Design review of the part built by this model. Coordinates are the model's own, in mm. A direction names the side the tool comes from. Coordinates: 2 decimals unless noted, no trailing zeros. Write each loop counter-clockwise with the first axis right and the second up, starting at its lowest first coordinate (ties: lowest second). Pieces come first, ordered by that corner, then holes.
Q1. Take a section at C-C (x = 5). Give the boundary of the cut face in (y, z).
Q2. Mouldability with a two-part tool opening along X and no side actions: class faces 6 (the flat face through (6.25, 0, 45)), 7 (the flat face through (10, 7, 13)), 8 (the flat face through (-19, 0, 30)), 9 (the flat face through (-7, 0, 12)) as pulls with the +X half, pulls with the -X half, needs draft (parallel to the pull), parting line crosses it, or undercut.
Q3. For probe 1 along X at (y, z) = (0, 24); probe 2 along Z at (x, y) = (4, 6); probe 3 along Y at (x, z) = (-3, 45), list the stretches that pass through material, from the lowest coordinate up.
Q4. Machinability: for faces 1 (the flat face through (19, 0, 30)), 2 (the flat face through (-25, 0, 35)), 3 (the flat face through (-6.25, 0, 45)), 4 (the flat face through (-11, 7, 12)), 5 (the flat face through (0, 3.5, 45)), which of the approach directions +Z, -Z, +X, -X, +Y, -Y give a long, thin tool a straight path to every point of the face, cutting with its end or side? Answer none if there is none.
Q5. Insertion check: pin 1 (6 mm diameter, centred on y = 1.5, z = 24.5, fed in from -X); pin 2 (7 mm diameter, centred on y = 0.5, z = 9.5, fed in from +X); pin 3 (2 mm diameter, centred on x = 4, y = -5.5, fed in from +Z). Each pin has a flat end and moves straight along its axis. Give the tip position at first contact, or say it passes through.
Q6. Take a section at B-B (y = -0.75). Give the boundary of the cut face in (x, z).
Q7. Take a section at A-A (z = 19). Give the boundary of the cut face in (x, y).
Q8. Take a section at D-D (z = 27). Give the boundary of the cut face in (x, y).
```python
from build123d import *

# Parameters (mm, degrees)
F0_W     = 7
F0_H     = 14
F1_DEPTH = 25
F2_W     = 38
F2_H     = 16
F3_DEPTH = 10
F4_W     = 60
F4_H     = 14
F5_DEPTH = 5
F6_W     = 12.5
F6_H     = 7
F7_DEPTH = 10
F8_W     = 7
F8_H     = 14
F9_DEPTH = 25


with BuildPart() as f1:
    # F0 (on Top) → F1 (new body)
    with BuildSketch(Plane.XY):
        with Locations((-10.5, 0)):
            Rectangle(F0_W, F0_H)
    extrude(amount=F1_DEPTH)

    # F2 (on face) → F3 (join)
    with BuildSketch(Plane.XY.offset(25)):
        Rectangle(F2_W, F2_H)
    extrude(amount=F3_DEPTH)

    # F4 (on face) → F5 (join)
    with BuildSketch(Plane.XY.offset(35)):
        Rectangle(F4_W, F4_H)
    extrude(amount=F5_DEPTH)

    # F6 (on face) → F7 (join)
    with BuildSketch(Plane.XY.offset(40)):
        Rectangle(F6_W, F6_H)
    extrude(amount=F7_DEPTH)

    # F8 (on face) → F9 (join, through all)
    with BuildSketch(Plane(origin=(0, 0, 25), x_dir=(1, 0, 0), z_dir=(0, 0, -1))):
        with Locations((10.5, 0)):
            Rectangle(F8_W, F8_H)
    extrude(amount=F9_DEPTH)


solid = f1.part
```
Response:
1. outline: (-8, 25) - (8, 25) - (8, 35) - (7, 35) - (7, 40) - (3.5, 40) - (3.5, 50) - (-3.5, 50) - (-3.5, 40) - (-7, 40) - (-7, 35) - (-8, 35) - close
2. face 6: pulls with the +X half
2. face 7: needs draft
2. face 8: pulls with the -X half
2. face 9: undercut
3. probe 1: x = -14 to -7, 7 to 14
3. probe 2: z = 25 to 40
3. probe 3: y = -3.5 to 3.5
4. face 1: -Z, +X, +Y, -Y
4. face 2: -Z, -X, +Y, -Y
4. face 3: +Z, -X, +Y, -Y
4. face 4: -Z, +X, -X, +Y
4. face 5: +Z, +X, -X, +Y
5. pin 1: stops at x = -19
5. pin 2: stops at x = 14
5. pin 3: stops at z = 40
6. outline: (-30, 35) - (-19, 35) - (-19, 25) - (-14, 25) - (-14, 0) - (-7, 0) - (-7, 25) - (7, 25) - (7, 0) - (14, 0) - (14, 25) - (19, 25) - (19, 35) - (30, 35) - (30, 40) - (6.25, 40) - (6.25, 50) - (-6.25, 50) - (-6.25, 40) - (-30, 40) - close
7. outline: (-14, -7) - (-7, -7) - (-7, 7) - (-14, 7) - close; (7, -7) - (14, -7) - (14, 7) - (7, 7) - close
8. outline: (-19, -8) - (19, -8) - (19, 8) - (-19, 8) - close
